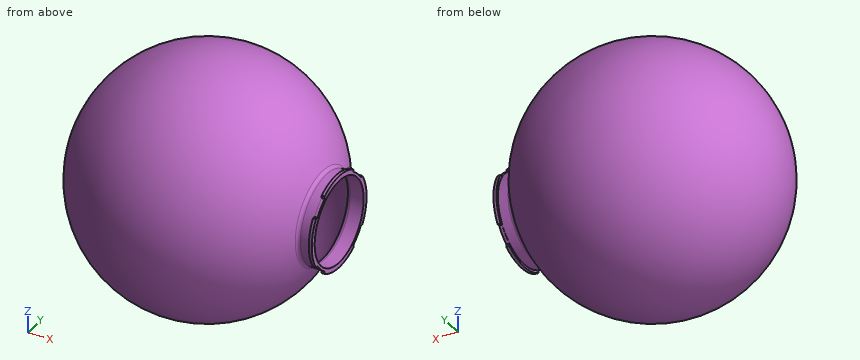
```python
from build123d import *

# Parameters (mm, degrees)
F3_DEPTH = 25


with BuildPart() as f1:
    # F0 (on Front) → F1 (revolve)
    with BuildSketch(Plane.XZ):
        with BuildLine():
            ThreePointArc((230.1764353028, -89.5980392157), (-45.581906938, -242.757677036), (-247, 0))
            Line((-247, 0), (-250, 0))
            ThreePointArc((-250, 0), (-48.1392607307, -245.3214454064), (231.4608926104, -94.476744186))
            ThreePointArc((231.4608926104, -94.476744186), (234.4059176567, -90.8597422297), (238.8676411739, -89.5))
            Line((238.8676411739, -89.5), (258.6609246731, -89.5))
            Line((258.6609246731, -89.5), (258.6609246731, -94.5))
            Line((258.6609246731, -94.5), (264.6609246731, -94.5))
            Line((264.6609246731, -94.5), (264.6609246731, -84.5))
            Line((264.6609246731, -84.5), (237.6315425191, -84.5))
            ThreePointArc((237.6315425191, -84.5), (233.1157749362, -85.8963765146), (230.1764353028, -89.5980392157))
        make_face()
    revolve(axis=Axis((132.3304623365, 0, 0), (1, 0, 0)))

    # F2 (on face) → F3 (cut)
    with BuildSketch(Plane.YZ.offset(264.6609246731)):
        with BuildLine():
            ThreePointArc((50, 74.8331477355), (63.6396103068, 63.6396103068), (74.8331477355, 50))
            Line((74.8331477355, 50), (80.1888396225, 50))
            ThreePointArc((80.1888396225, 50), (66.8215908221, 66.8215908221), (50, 80.1888396225))
            Line((50, 80.1888396225), (50, 74.8331477355))
        make_face()
        with BuildLine():
            Line((80.1888396225, -50), (74.8331477355, -50))
            ThreePointArc((74.8331477355, -50), (63.6396103068, -63.6396103068), (50, -74.8331477355))
            Line((50, -74.8331477355), (50, -80.1888396225))
            ThreePointArc((50, -80.1888396225), (66.8215908221, -66.8215908221), (80.1888396225, -50))
        make_face()
        with BuildLine():
            Line((119.5877417922, 50), (80.1888396225, 50))
            ThreePointArc((80.1888396225, 50), (90.8517895925, 26.0038906289), (94.5, 0))
            ThreePointArc((94.5, 0), (90.8517895925, -26.0038906289), (80.1888396225, -50))
            Line((80.1888396225, -50), (119.5877417922, -50))
            Line((119.5877417922, -50), (119.5877417922, 50))
        make_face()
        with BuildLine():
            ThreePointArc((-74.8331477355, 50), (-63.6396103068, 63.6396103068), (-50, 74.8331477355))
            Line((-50, 74.8331477355), (-50, 80.1888396225))
            ThreePointArc((-50, 80.1888396225), (-66.8215908221, 66.8215908221), (-80.1888396225, 50))
            Line((-80.1888396225, 50), (-74.8331477355, 50))
        make_face()
        with BuildLine():
            Line((-50, -80.1888396225), (-50, -74.8331477355))
            ThreePointArc((-50, -74.8331477355), (-63.6396103068, -63.6396103068), (-74.8331477355, -50))
            Line((-74.8331477355, -50), (-80.1888396225, -50))
            ThreePointArc((-80.1888396225, -50), (-66.8215908221, -66.8215908221), (-50, -80.1888396225))
        make_face()
        with BuildLine():
            ThreePointArc((-80.1888396225, -50), (-94.5, 0), (-80.1888396225, 50))
            Line((-80.1888396225, 50), (-119.5877417922, 50))
            Line((-119.5877417922, 50), (-119.5877417922, -50))
            Line((-119.5877417922, -50), (-80.1888396225, -50))
        make_face()
    extrude(amount=-F3_DEPTH, mode=Mode.SUBTRACT)


solid = f1.part
```
For this review, take the finished solid that the model builds, in its own axes (mm). Round coordinates to 2 decimals unless told otherwise and drop trailing zeros. Order: outer loops, then holes, each group sorted by start corner. A loop starts at its lowest first (then second) coordinate and runs counter-clockwise, first axis right, second up.
Q1. We need section A-A, the plane y = 0. Give the boundary of the cut face in (x, z).
Findings below:
outline: (230.18, -89.6) arc R247 cw (long way) to (230.18, 89.6) arc R8 ccw to (237.63, 84.5) - (264.66, 84.5) - (264.66, 94.5) - (258.66, 94.5) - (258.66, 89.5) - (238.87, 89.5) arc R8 cw to (231.46, 94.48) arc R250 ccw (long way) to (231.46, -94.48) arc R8 cw to (238.87, -89.5) - (258.66, -89.5) - (258.66, -94.5) - (264.66, -94.5) - (264.66, -84.5) - (237.63, -84.5) arc R8 ccw to start
Q2. We need section C-C, the plane z = 202. Give the boundary of the cut face in (x, y), plus the area to 3 significant figures.
Findings below:
outline: circle Ø294.59 at (0, 0); hole circle Ø284.29 at (0, 0)
area: 4,680 mm2
Q3. Wall thickness on line 1 (Y direction, x = 248.75, z = 0); line 2 (Z direction, x = 211.5, y = 52.5); line 3 (X direction, y = -80, z = -40): over which ranges is each line inside the solid? List them lowest first.
Findings below:
line 1: y = -89.5 to -84.5, 84.5 to 89.5
line 2: z = -122.52 to -116.28, 116.28 to 122.52
line 3: x = -233.45 to -230.24, 230.24 to 264.66
Q4. Insertion check: P1, Ø1.6, axis at x = 261.5, y = -77, coming from the -Z side; P2, Ø1.5, axis at x = 16.5, z = 155.5, coming from the +Y side; P3, Ø10, axis at x = -195, y = -21.5, coming from the +Z side; P4, Ø1, axis at x = 174.5, z = 181, coming from the -Y side. Each pin has a flat end and moves straight along its axis. Give the tip position at first contact, or say it passes through.
Findings below:
P1: stops at z = -50
P2: stops at y = 195.66
P3: stops at z = 161.09
P4: passes through
Q5. We need section D-D, the plane x = 0.5. Give the boundary of the cut face in (y, z).
Findings below:
outline: circle Ø500 at (0, 0); hole circle Ø494 at (0, 0)
